Check sheet for the drawn part. Datum: minimum x, y, z corner. Units: mm. Round coordinates to 2 decimals unless told otherwise and drop trailing zeros. Write each loop counter-clockwise with the first axis right and the second up, starting at its lowest first coordinate (ties: lowest second). Pieces come first, ordered by that corner, then holes.
Item 1: Cross-section at D-D on y = 2.15. Enter the section's corners in (x, z).
Item 2: Cross-section at C-C on z = 5. Enter the section's corners in (x, y), plus the area to 3 significant figures.
Item 3: Cross-section at B-B on z = 27. Enter the section's corners in (x, y), plus the area to 3 significant figures.
Item 4: Material ranges on line 1 (Z direction, x = 55, y = 2.1); line 2 (Z direction, x = 54, y = 1.65); line 3 (Z direction, x = 35, y = 1.15), recorded low to high.
Item 5: Cross-section at A-A on x = 55. Enter the section's corners in (y, z).
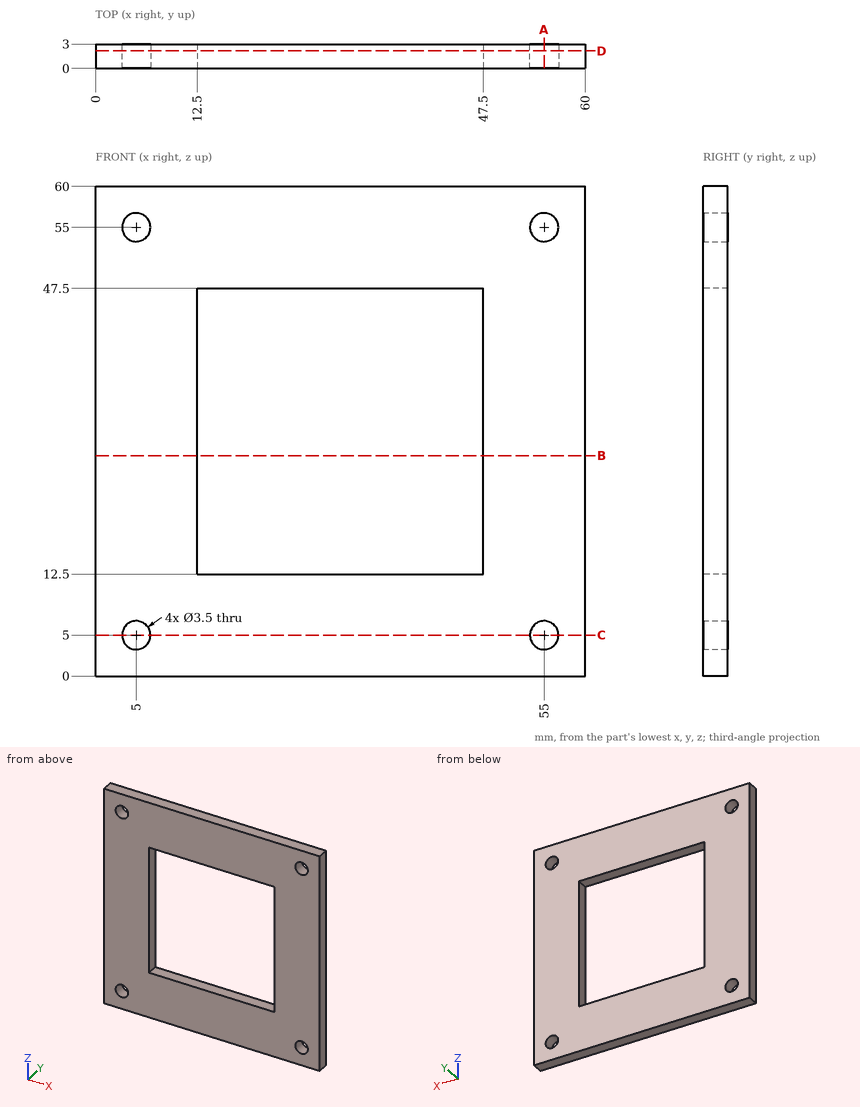
Response values:
1. outline: (0, 0) - (60, 0) - (60, 60) - (0, 60) - close; hole circle Ø3.5 at (5, 5); hole circle Ø3.5 at (5, 55); hole (12.5, 12.5) - (47.5, 12.5) - (47.5, 47.5) - (12.5, 47.5) - close; hole circle Ø3.5 at (55, 5); hole circle Ø3.5 at (55, 55)
2. outline: (0, 0) - (3.25, 0) - (3.25, 3) - (0, 3) - close; (6.75, 0) - (53.25, 0) - (53.25, 3) - (6.75, 3) - close; (56.75, 0) - (60, 0) - (60, 3) - (56.75, 3) - close
2. area: 159 mm2
3. outline: (0, 0) - (12.5, 0) - (12.5, 3) - (0, 3) - close; (47.5, 0) - (60, 0) - (60, 3) - (47.5, 3) - close
3. area: 75.0 mm2
4. line 1: z = 0 to 3.25, 6.75 to 53.25, 56.75 to 60
4. line 2: z = 0 to 3.56, 6.44 to 53.56, 56.44 to 60
4. line 3: z = 0 to 12.5, 47.5 to 60
5. outline: (0, 0) - (3, 0) - (3, 3.25) - (0, 3.25) - close; (0, 6.75) - (3, 6.75) - (3, 53.25) - (0, 53.25) - close; (0, 56.75) - (3, 56.75) - (3, 60) - (0, 60) - close
